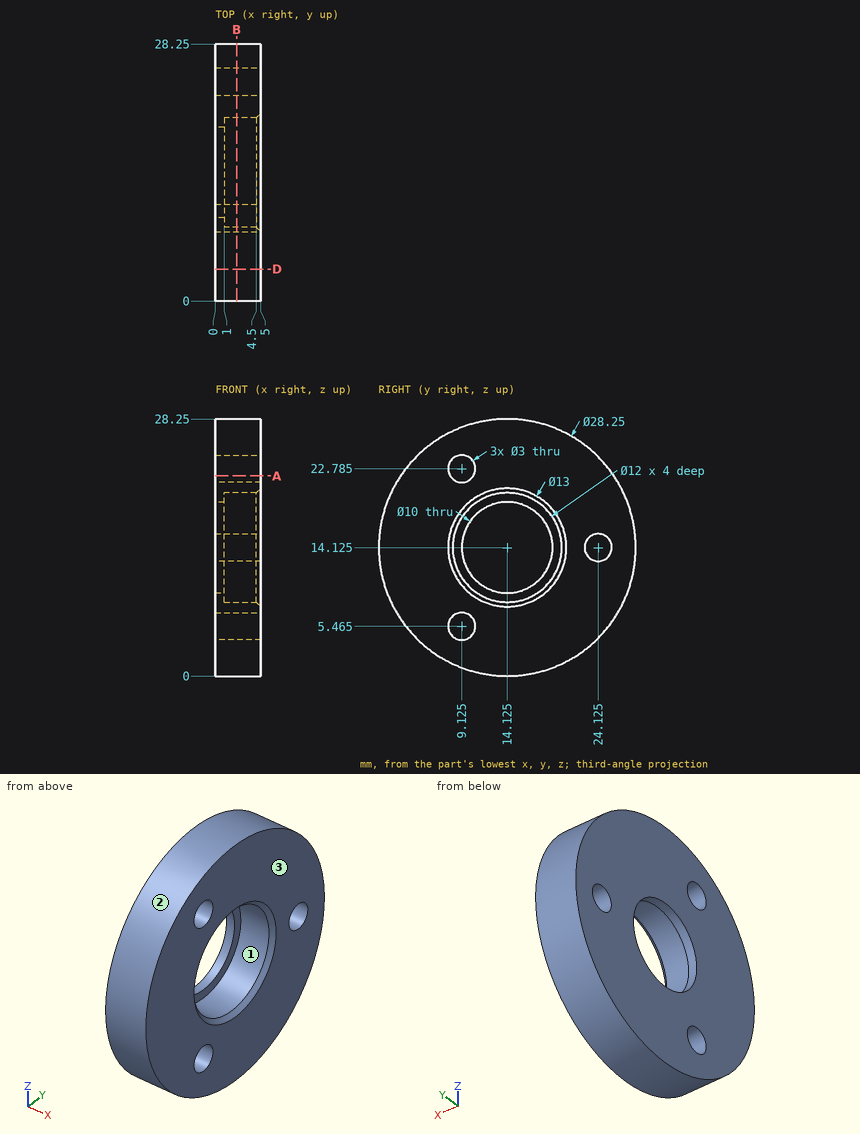
Print and shaded views of the part. All mm, measured from the part's lowest x, y and z. Give positions to 0.01 mm unless a question says otherwise; leave off trailing zeros. Loops run counter-clockwise (first coordinate to the right, second up) from the corner with the lowest first, then second, coordinate; pieces in that order, holes last. Notation, with made-up numbers: (1.5, -21.75) -> (7.5, -21.75) arc R28 ccw to (7.5, 14.25) -> close; hole circle Ø1 at (3, 37). An arc over 180 degrees is marked (long way). One line per question, with ' | ' between items. Start each with the question number.
1) Two-plate mould, pull along Z, no slides. Class the marked faces 1, 2 and 3: released by +Z, released by -Z, zero draft, split by the parting line, or undercut.
2) Cut at B-B (x = 2.35). Count the separate pieces of the cut face and the enclosed holes in it.
3) Pin check, flat tips, straight feed: pin 1 (9.5 mm diameter, centred on y = 13.5, z = 14, fed in from +X); pin 2 (1.8 mm diameter, centred on y = 9.12, z = 5.46, fed in from +X). Stop position of each tip, or through.
4) Cut at A-A (z = 22). Give the cut face in (x, y).
5) Cut at D-D (y = 3.5). Give the cut face in (x, z).
6) Probe L1, parallel to Y at x = 1.95, z = 13.5; L2, parallel to Y at x = 3.75, z = 14.5 (1 decimal); L3, parallel to Z at x = 2.1, y = 8. List the from-to ranges inside material, lowest first.
Return value:
1) face 1: undercut | face 2: split by the parting line | face 3: zero draft
2) separate pieces: 1 | enclosed holes: 4
3) pin 1: x = 1 | pin 2: through
4) outline: (0, 2.4) -> (5, 2.4) -> (5, 7.85) -> (0, 7.85) -> close; (0, 10.4) -> (5, 10.4) -> (5, 25.85) -> (0, 25.85) -> close
5) outline: (0, 4.82) -> (5, 4.82) -> (5, 23.43) -> (0, 23.43) -> close
6) L1: 0.01 to 8.16, 20.09 to 22.76, 25.49 to 28.24 | L2: 0 to 8.1, 20.1 to 22.7, 25.6 to 28.2 | L3: 1.4 to 4.47, 6.46 to 21.79, 23.78 to 26.85
